from build123d import *

# Parameters (mm, degrees)
F0_W     = 50
F0_H     = 32
F1_DEPTH = 2.5
F2_R     = 2.5
F3_SIZE2 = 2.49999
F3_SIZE  = 1.750509


# Not quite as in the source:
# - a fillet or chamfer is up to 0.001 mm smaller than in the source, because OpenCascade refuses the exact size


with BuildPart() as f1:
    # F0 (on Top) → F1 (new body)
    with BuildSketch(Plane.XY):
        Rectangle(F0_W, F0_H)
    extrude(amount=F1_DEPTH)

    # F2
    f2_edges = [f1.edges().sort_by_distance(p)[0] for p in [
        (-25, -16, 1.25),
        (25, -16, 1.25),
        (25, 16, 1.25),
        (-25, 16, 1.25),
    ]]
    fillet(f2_edges, radius=F2_R)

    # F3 (size 1.7505188455 and 2.5 in the source; OpenCascade refuses exactly that, so slightly less here)
    f3_edges = [f1.edges().sort_by_distance(p)[0] for p in [
        (0, -16, 2.5),
        (-24.267767, -15.267767, 2.5),
        (-25, 0, 2.5),
        (-24.267767, 15.267767, 2.5),
        (0, 16, 2.5),
        (24.267767, 15.267767, 2.5),
        (25, 0, 2.5),
        (24.267767, -15.267767, 2.5),
    ]]
    f3_side = f1.faces().sort_by_distance((0, 0, 2.5))[0]
    chamfer(f3_edges, length=F3_SIZE, length2=F3_SIZE2, reference=f3_side)


solid = f1.part
The model under review builds one solid part; all positions refer to its coordinate system, in mm. Coordinates: 2 decimals unless noted, no trailing zeros. Write each loop counter-clockwise with the first axis right and the second up, starting at its lowest first coordinate (ties: lowest second). Pieces come first, ordered by that corner, then holes. Notation, with made-up numbers: (-5.5, 15.5) - (41.5, 15.5) arc R30 cw to (41.5, 46.5) - close; hole circle Ø2 at (7, 14). An arc over 180 degrees is marked (long way). Answer as a JSON object with one key per item and string values. Group by question number.
1. Clearance check with flat-ended pins moving along their axes: pin 1 Ø1.5 at (x, z) = (5.5, 1) entering from +Y; pin 2 Ø1 at (x, z) = (-10, 2) entering from +Y. State where each tip first meets the part, or that it passes through.
2. To check wall thickness, follow probe 1 along Y at (x, z) = (5.5, 1.25); probe 2 along X at (y, z) = (2, 0.25); probe 3 along Y at (x, z) = (15, 0.65). State the ranges of each line that lie inside material, in increasing order.
3. Add section C-C (z = 0.4). Give the boundary of the cut face in (x, y), plus the area to 3 significant figures.
Findings:
{
 "1": {"pin 1": "y = 15.82", "pin 2": "y = 14.95"},
 "2": {"probe 1": "-15.12 to 15.12", "probe 2": "-24.82 to 24.82", "probe 3": "-15.54 to 15.54"},
 "3": {"outline": "(-24.72, -13.5) arc R2.22 ccw to (-22.5, -15.72) - (22.5, -15.72) arc R2.22 ccw to (24.72, -13.5) - (24.72, 13.5) arc R2.22 ccw to (22.5, 15.72) - (-22.5, 15.72) arc R2.22 ccw to (-24.72, 13.5) - close", "area": "1,550 mm²"}
}
